The drawing under review shows one solid part. Ordinate dimensions are in mm from its lowest x, y, z. A direction names the side the tool comes from. Coordinates: 2 decimals unless noted, no trailing zeros. Order: outer loops, then holes, each group sorted by start corner. A loop starts at its lowest first (then second) coordinate and runs counter-clockwise, first axis right, second up. Notation, with made-up numbers: (86.5, 79) - (131.5, 79) arc R32 ccw to (131.5, 113) - close; hole circle Ø11 at (28.5, 12). An arc over 180 degrees is marked (long way). Answer in a Markdown table with one row per item.
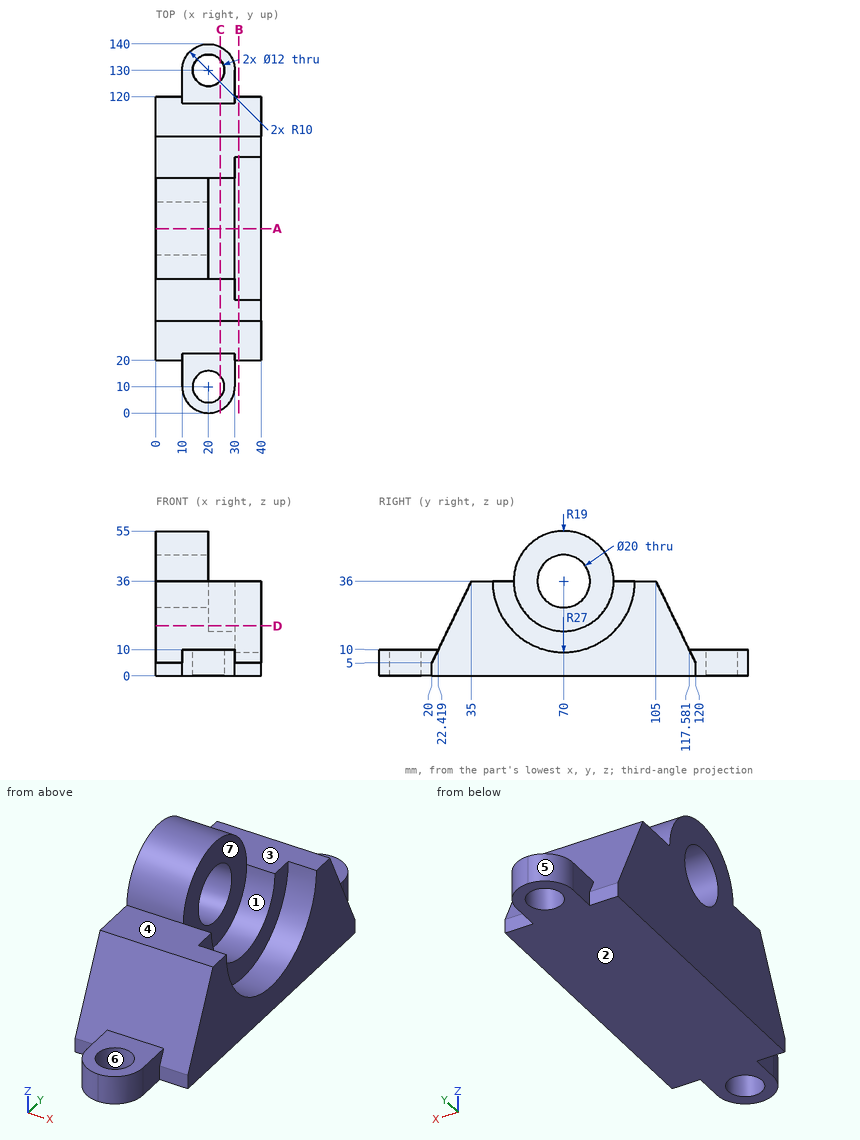
Item 1: We need section C-C, the plane x = 24.5. Write out the cut boundary in (y, z), then the cut area to 3 significant figures.
Check values:
| item | result |
|---|---|
| outline | (1.07, 0) - (6.03, 0) - (6.03, 10) - (1.07, 10) - close; (13.97, 0) - (126.03, 0) - (126.03, 10) - (117.58, 10) - (105, 36) - (89, 36) arc R19 cw to (51, 36) - (35, 36) - (22.42, 10) - (13.97, 10) - close; (133.97, 0) - (138.93, 0) - (138.93, 10) - (133.97, 10) - close |
| area | 2,800 mm^2 |
Item 2: Mouldability with a two-part tool opening along X and no side actions: class the marked faces 5, 6 and 7 as +X half, -X half, draft (parallel to the pull), parting line (faces both ways), or undercut.
Check values:
| item | result |
|---|---|
| face 5 | -X half |
| face 6 | undercut |
| face 7 | +X half |
Item 3: To check wall thickness, follow line 1 (Z direction, x = 14.5, y = 46.5); line 2 (Z direction, x = 14, y = 70); line 3 (Y direction, x = 3.5, z = 10). State the ranges of each line that lie inside material, in increasing order. Write a range as from..to.
Check values:
| item | result |
|---|---|
| line 1 | 0..36 |
| line 2 | 0..26, 46..55 |
| line 3 | 22.42..117.58 |
Item 4: We need section D-D, the plane z = 19. Write out the cut boundary in (x, y) (1 decimal), then the cut area to 3 significant figures.
Check values:
| item | result |
|---|---|
| outline | (0, 26.8) - (40, 26.8) - (40, 49) - (30, 49) - (30, 61.5) - (20, 61.5) - (20, 78.5) - (30, 78.5) - (30, 91) - (40, 91) - (40, 113.2) - (0, 113.2) - close |
| area | 2,870 mm^2 |
Item 5: We need section B-B, the plane x = 31.5. Write out the cut boundary in (y, z).
Check values:
| item | result |
|---|---|
| outline | (20, 0) - (120, 0) - (120, 5) - (105, 36) - (97, 36) arc R27 cw to (43, 36) - (35, 36) - (20, 5) - close |
Item 6: We need section A-A, the plane y = 70. Write out the cut boundary in (x, z).
Check values:
| item | result |
|---|---|
| outline | (0, 0) - (40, 0) - (40, 9) - (30, 9) - (30, 17) - (20, 17) - (20, 26) - (0, 26) - close; (0, 46) - (20, 46) - (20, 55) - (0, 55) - close |
Item 7: Tool access review of the marked faces 1, 2, 3 and 4: name each direction out of +Z, -Z, +X, -X, +Y, -Y from which nothing blocks a thin tool from reaching the whole face with its end or side.
Check values:
| item | result |
|---|---|
| face 1 | +Z, +X |
| face 2 | -Z, +X, -X, +Y, -Y |
| face 3 | +Z, +X, -X, +Y |
| face 4 | +Z, +X, -X, -Y |
Item 8: Clearance check with flat-ended pins moving along their axes: pin 1 Ø1 at (x, y) = (34, 69) entering from +Z; pin 2 Ø1.5 at (x, y) = (13.5, 78) entering from +Z; pin 3 Ø5 at (y, z) = (17, 3.5) entering from +X; pin 4 Ø6 at (x, y) = (20, 132) entering from +Z. State where each tip first meets the part, or that it passes through.
Check values:
| item | result |
|---|---|
| pin 1 | z = 9.04 |
| pin 2 | z = 53.56 |
| pin 3 | x = 30 |
| pin 4 | through |
